```python
from build123d import *

# Parameters (mm, degrees)
SKETCH_2_W          = 119
SKETCH_2_H          = 120
EXTRUDE_1_DEPTH     = 2
SKETCH_6_R          = 2
CUT_EXTRUDE_3_DEPTH = 2
CUT_EXTRUDE_5_DEPTH = 2
FILLET_1_R          = 2
SKETCH_9_R          = 2
CUT_EXTRUDE_6_DEPTH = 2


with BuildPart() as part:
    # 草图2 → 凸台-拉伸1 (new body)
    with BuildSketch(Plane.XY):
        with Locations((59.5, 60)):
            Rectangle(SKETCH_2_W, SKETCH_2_H)
    extrude(amount=EXTRUDE_1_DEPTH)

    # 草图6 → 切除-拉伸3 (cut)
    with BuildSketch(Plane.XY):
        with Locations((8.5, 100)):
            Circle(SKETCH_6_R)
        with Locations((30.5, 100)):
            Circle(SKETCH_6_R)
        with Locations((8.5, 87)):
            Circle(SKETCH_6_R)
        with Locations((30.5, 87)):
            Circle(SKETCH_6_R)
        with Locations((54, 93.5)):
            Circle(SKETCH_6_R)
        with Locations((88.5, 100)):
            Circle(SKETCH_6_R)
        with Locations((88.5, 87)):
            Circle(SKETCH_6_R)
        with Locations((110.5, 100)):
            Circle(SKETCH_6_R)
        with Locations((110.5, 87)):
            Circle(SKETCH_6_R)
        with Locations((88.5, 74)):
            Circle(SKETCH_6_R)
        with Locations((88.5, 61)):
            Circle(SKETCH_6_R)
        with Locations((110.5, 74)):
            Circle(SKETCH_6_R)
        with Locations((110.5, 61)):
            Circle(SKETCH_6_R)
    extrude(amount=CUT_EXTRUDE_3_DEPTH, mode=Mode.SUBTRACT)

    # 草图7 → 切除-拉伸5 (cut)
    with BuildSketch(Plane.XY):
        with BuildLine():
            ThreePointArc((59.618141264, 81.233145737), (64.538696872, 86.493844671), (66.498605851, 93.425336399))
            ThreePointArc((66.498605851, 93.425336399), (64.574663601, 95.498605851), (62.501394149, 93.574663601))
            ThreePointArc((62.501394149, 93.574663601), (61.055127678, 88.459740312), (57.424125079, 84.577737339))
            ThreePointArc((57.424125079, 84.577737339), (56.848837371, 81.808433446), (59.618141264, 81.233145737))
        make_face()
    extrude(amount=CUT_EXTRUDE_5_DEPTH, mode=Mode.SUBTRACT)

    # 圆角1
    fillet_1_edges = [part.edges().sort_by_distance(p)[0] for p in [
        (0, 0, 1),
        (119, 0, 1),
        (119, 120, 1),
        (0, 120, 1),
    ]]
    fillet(fillet_1_edges, radius=FILLET_1_R)

    # 草图9 → 切除-拉伸6 (cut)
    with BuildSketch(Plane.XY.offset(2)):
        with Locations((4, 116)):
            Circle(SKETCH_9_R)
        with Locations((115, 116)):
            Circle(SKETCH_9_R)
        with Locations((4, 4)):
            Circle(SKETCH_9_R)
        with Locations((115, 4)):
            Circle(SKETCH_9_R)
    extrude(amount=-CUT_EXTRUDE_6_DEPTH, mode=Mode.SUBTRACT)


solid = part.part
```
Model file for the job. Use its own axes, mm. Coordinates: 2 decimals unless noted, no trailing zeros. Loops run counter-clockwise (first coordinate to the right, second up) from the corner with the lowest first, then second, coordinate; pieces in that order, holes last. Notation, with made-up numbers: (69.25, 65) - (115.25, 65) arc R17 ccw to (115.25, 79) - close; hole circle Ø4 at (50.25, 33). An arc over 180 degrees is marked (long way). Answer as a JSON object with one key per item and string values. Group by question number.
(1) Probe line 1 along Y through (x, z) = (110.5, 0.9); line 2 along Y through (x, z) = (4, 0.55); line 3 along Y through (x, z) = (30.5, 0.5). List the from-to ranges inside material, lowest first.
(2) Two-plate mould, pull along Y, no slides. Class faces 1 (the face through (59, 61, 0)), 2 (the face through (89.575, 101.686, 0.986)), 3 (the face through (90.408, 61.601, 0.986)): released by +Y, released by -Y, zero draft, split by the parting line, or undercut.
(3) Cut at D-D (z = 0.95). State how many separate pieces and enclosed holes the cut face has, then the cut area to 3 significant figures.
(4) Cut at B-B (x = 54). Give the cut face in (y, z).
(5) Cut at A-A (y = 61). Give the cut face in (x, z).
(6) Cut at C-C (x = 8.5). Give the cut face in (y, z), then the cut area to 3 significant figures.
Geometry says:
{
 "1": {"line 1": "y = 0 to 59, 63 to 72, 76 to 85, 89 to 98, 102 to 120", "line 2": "y = 0 to 2, 6 to 114, 118 to 120", "line 3": "y = 0 to 85, 89 to 98, 102 to 120"},
 "2": {"face 1": "zero draft", "face 2": "undercut", "face 3": "undercut"},
 "3": {"separate pieces": "1", "enclosed holes": "18", "area": "14,000 mm^2"},
 "4": {"outline": "(0, 0) - (91.5, 0) - (91.5, 2) - (0, 2) - close; (95.5, 0) - (120, 0) - (120, 2) - (95.5, 2) - close"},
 "5": {"outline": "(0, 0) - (86.5, 0) - (86.5, 2) - (0, 2) - close; (90.5, 0) - (108.5, 0) - (108.5, 2) - (90.5, 2) - close; (112.5, 0) - (119, 0) - (119, 2) - (112.5, 2) - close"},
 "6": {"outline": "(0, 0) - (85, 0) - (85, 2) - (0, 2) - close; (89, 0) - (98, 0) - (98, 2) - (89, 2) - close; (102, 0) - (120, 0) - (120, 2) - (102, 2) - close", "area": "224 mm^2"}
}
